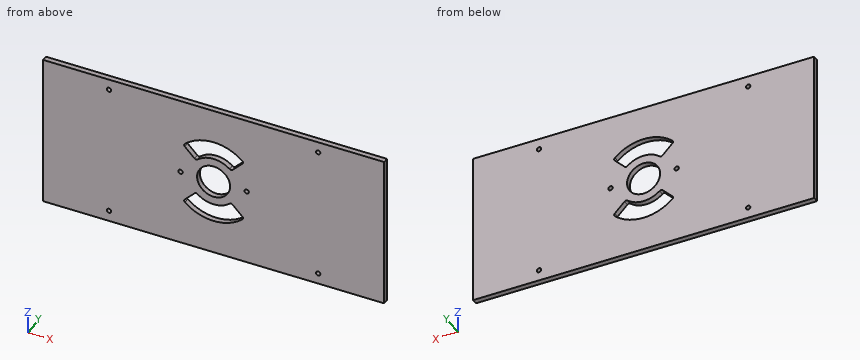
from build123d import *

# Parameters (mm, degrees)
SKETCH2_W           = 310
SKETCH2_H           = 140
BOSS_EXTRUDE1_DEPTH = 5
SKETCH3_R           = 15
CUT_EXTRUDE1_DEPTH  = 6
SKETCH5_R           = 2
CUT_EXTRUDE2_DEPTH  = 6
CUT_EXTRUDE3_DEPTH  = 10
FILLET1_R           = 2
SKETCH7_R           = 2
CUT_EXTRUDE4_DEPTH  = 6


with BuildPart() as part:
    # Sketch2 → Boss-Extrude1 (new body)
    with BuildSketch(Plane(origin=(0, 0, 0), x_dir=(1, 0, 0), z_dir=(0, 1, 0))):
        Rectangle(SKETCH2_W, SKETCH2_H)
    extrude(amount=BOSS_EXTRUDE1_DEPTH)

    # Sketch3 → Cut-Extrude1 (cut, through all)
    with BuildSketch(Plane(origin=(0, 5, 0), x_dir=(1, 0, 0), z_dir=(0, 1, 0))):
        Circle(SKETCH3_R)
    extrude(amount=-CUT_EXTRUDE1_DEPTH, mode=Mode.SUBTRACT)

    # Sketch5 → Cut-Extrude2 (cut, through all)
    with BuildSketch(Plane(origin=(0, 5, 0), x_dir=(1, 0, 0), z_dir=(0, 1, 0))):
        with Locations((-95, 60)):
            Circle(SKETCH5_R)
        with Locations((95, 60)):
            Circle(SKETCH5_R)
        with Locations((95, -60)):
            Circle(SKETCH5_R)
        with Locations((-95, -60)):
            Circle(SKETCH5_R)
    extrude(amount=-CUT_EXTRUDE2_DEPTH, mode=Mode.SUBTRACT)

    # Sketch6 → Cut-Extrude3 (cut)
    with BuildSketch(Plane(origin=(0, 5, 0), x_dir=(1, 0, 0), z_dir=(0, 1, 0))):
        with BuildLine():
            Line((27.577164466, -27.577164466), (15.909902577, -15.909902577))
            ThreePointArc((15.909902577, -15.909902577), (0, -22.5), (-15.909902577, -15.909902577))
            Line((-15.909902577, -15.909902577), (-27.577164466, -27.577164466))
            ThreePointArc((-27.577164466, -27.577164466), (0, -39), (27.577164466, -27.577164466))
        make_face()
        with BuildLine():
            ThreePointArc((-15.909902577, 15.909902577), (0, 22.5), (15.909902577, 15.909902577))
            Line((15.909902577, 15.909902577), (27.577164466, 27.577164466))
            ThreePointArc((27.577164466, 27.577164466), (0, 39), (-27.577164466, 27.577164466))
            Line((-27.577164466, 27.577164466), (-15.909902577, 15.909902577))
        make_face()
    extrude(amount=-CUT_EXTRUDE3_DEPTH, mode=Mode.SUBTRACT)

    # Fillet1
    fillet1_edges = [part.edges().sort_by_distance(p)[0] for p in [
        (-15.909902577, 2.5, 15.909902577),
        (15.909902577, 2.5, 15.909902577),
        (27.577164466, 2.5, 27.577164466),
        (-27.577164466, 2.5, 27.577164466),
        (15.909902577, 2.5, -15.909902577),
        (-15.909902577, 2.5, -15.909902577),
        (-27.577164466, 2.5, -27.577164466),
        (27.577164466, 2.5, -27.577164466),
    ]]
    fillet(fillet1_edges, radius=FILLET1_R)

    # Sketch7 → Cut-Extrude4 (cut, through all)
    with BuildSketch(Plane(origin=(0, 5, 0), x_dir=(1, 0, 0), z_dir=(0, 1, 0))):
        with Locations((-30, 0)):
            Circle(SKETCH7_R)
        with Locations((30, 0)):
            Circle(SKETCH7_R)
    extrude(amount=-CUT_EXTRUDE4_DEPTH, mode=Mode.SUBTRACT)


solid = part.part
CAD build for the part. Positions are in the model's coordinates, mm. Round coordinates to 2 decimals unless told otherwise and drop trailing zeros. Order: outer loops, then holes, each group sorted by start corner. A loop starts at its lowest first (then second) coordinate and runs counter-clockwise, first axis right, second up. Notation, with made-up numbers: (55, 80.25) -> (62, 80.25) arc R24 ccw to (62, 118.25) -> close; hole circle Ø7 at (0.25, -17.75). An arc over 180 degrees is marked (long way). Write item = value, one per line. Start each with the question number.
(1) Cut at C-C, the plane z = 33. List the corners of the cut face in (x, y), then the cut area to 3 significant figures.
(2) Cut at B-B, the plane y = 1. State how many separate pieces and enclosed holes the cut face has, then the cut area to 3 significant figures.
(3) Cut at A-A, the plane x = 0. List the corners of the cut face in (y, z), then the cut area to 3 significant figures.
(4) Probe line 1 (X direction, y = 2.25, z = -60); line 2 (X direction, y = 3.8, z = 0); line 3 (Z direction, x = 95, y = 1.5). List the from-to ranges inside material, lowest first. Write a range as [from, to].
Model answer:
q1.outline = (-155, 0) -> (-20.78, 0) -> (-20.78, 5) -> (-155, 5) -> close; (20.78, 0) -> (155, 0) -> (155, 5) -> (20.78, 5) -> close
q1.area = 1,340 mm2
q2.separate_pieces = 1
q2.enclosed_holes = 9
q2.area = 41,000 mm2
q3.outline = (0, -70) -> (5, -70) -> (5, -39) -> (0, -39) -> close; (0, -22.5) -> (5, -22.5) -> (5, -15) -> (0, -15) -> close; (0, 15) -> (5, 15) -> (5, 22.5) -> (0, 22.5) -> close; (0, 39) -> (5, 39) -> (5, 70) -> (0, 70) -> close
q3.area = 385 mm2
q4.line_1 = [-155, -97], [-93, 93], [97, 155]
q4.line_2 = [-155, -32], [-28, -15], [15, 28], [32, 155]
q4.line_3 = [-70, -62], [-58, 58], [62, 70]
